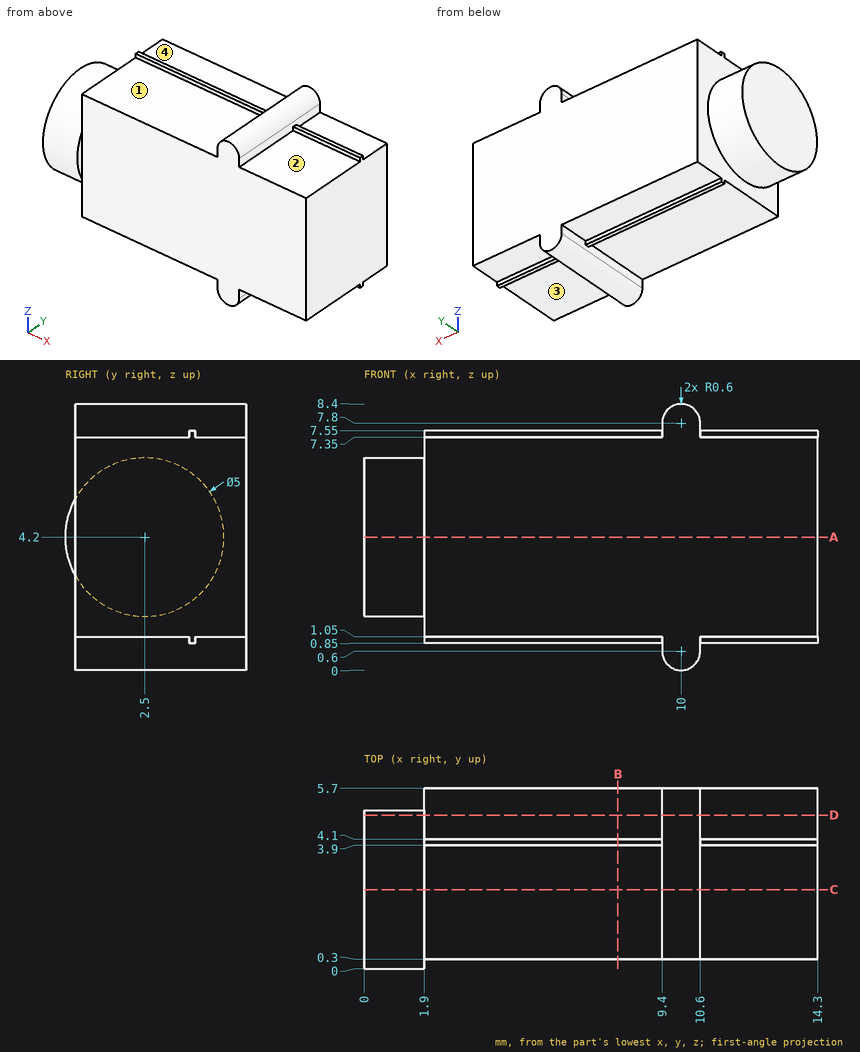
Drawing for the job (mm, zero at the part's lowest x, y, z). A direction names the side the tool comes from. Round coordinates to 2 decimals unless told otherwise and drop trailing zeros. Loops run counter-clockwise (first coordinate to the right, second up) from the corner with the lowest first, then second, coordinate; pieces in that order, holes last. Notation, with made-up numbers: (44.25, 17.25) - (49.25, 17.25) arc R21 ccw to (49.25, 54.25) - close; hole circle Ø9 at (46.25, 26). An arc over 180 degrees is marked (long way). Return JSON: item names as keys, results as strings. Group by question number.
Q1. Band-saw the part on C-C on y = 2.5. Give the cut face in (x, z), plus the area to 3 significant figures.
Q2. Drill centre lines: line 1 along X through (y, z) = (3.95, 6.75); line 2 along Z through (x, y) = (3, 2.1); line 3 along Y through (x, z) = (7.5, 3). Where is each one in solid material? Low to high. Write a range as [from, to].
Q3. Band-saw the part on D-D on y = 4.85. Give the cut face in (x, z).
Q4. Flat gauge pins, fed straight in: pin 1 Ø1.8 at (x, y) = (12.5, 2.5) entering from -Z; pin 2 Ø2 at (x, z) = (9, 3.5) entering from -Y; pin 3 Ø1.1 at (x, y) = (6, 2) entering from +Z. Where does each tip first touch, or does it go through?
Q5. Band-saw the part on B-B on x = 8. Give the cut face in (y, z), plus the area to 3 significant figures.
Q6. Tool access for the marked faces 1, 2, 3 and 4: list every direction of +Z, -Z, +X, -X, +Y, -Y with a clear straight run to the whole face (end or side of a thin tool).
Q7. Band-saw the part on A-A on z = 4.2. Give the cut face in (x, y).
Solutions:
{
 "1": {"outline": "(0, 1.7) - (1.9, 1.7) - (1.9, 1.05) - (9.4, 1.05) - (9.4, 0.6) arc R0.6 ccw to (10.6, 0.6) - (10.6, 1.05) - (14.3, 1.05) - (14.3, 7.35) - (10.6, 7.35) - (10.6, 7.8) arc R0.6 ccw to (9.4, 7.8) - (9.4, 7.35) - (1.9, 7.35) - (1.9, 6.7) - (0, 6.7) - close", "area": "89.8 mm^2"},
 "2": {"line 1": "x = [1.9, 14.3]", "line 2": "z = [1.05, 7.35]", "line 3": "y = [0.3, 5.7]"},
 "3": {"outline": "(0, 3.35) - (1.9, 3.35) - (1.9, 1.05) - (9.4, 1.05) - (9.4, 0.6) arc R0.6 ccw to (10.6, 0.6) - (10.6, 1.05) - (14.3, 1.05) - (14.3, 7.35) - (10.6, 7.35) - (10.6, 7.8) arc R0.6 ccw to (9.4, 7.8) - (9.4, 7.35) - (1.9, 7.35) - (1.9, 5.05) - (0, 5.05) - close"},
 "4": {"pin 1": "stops at z = 1.05", "pin 2": "stops at y = 0.3", "pin 3": "stops at z = 7.35"},
 "5": {"outline": "(0.3, 1.05) - (3.9, 1.05) - (3.9, 0.85) - (4.1, 0.85) - (4.1, 1.05) - (5.7, 1.05) - (5.7, 7.35) - (4.1, 7.35) - (4.1, 7.55) - (3.9, 7.55) - (3.9, 7.35) - (0.3, 7.35) - close", "area": "34.1 mm^2"},
 "6": {"face 1": "+Z, -X, -Y", "face 2": "+Z, +X, -Y", "face 3": "-Z, +X, -Y", "face 4": "+Z, -X, +Y"},
 "7": {"outline": "(0, 0) - (1.9, 0) - (1.9, 0.3) - (14.3, 0.3) - (14.3, 5.7) - (1.9, 5.7) - (1.9, 5) - (0, 5) - close"}
}
